Verification items for the finished model (mm, model axes). Coordinates: 2 decimals unless noted, no trailing zeros. Order: outer loops, then holes, each group sorted by start corner. A loop starts at its lowest first (then second) coordinate and runs counter-clockwise, first axis right, second up. Notation, with made-up numbers: M -33.75,29 L 9.25,29 A9 ccw 9.25,45 Z; hole C -31,-10 d3. An arc over 180 degrees is marked long. Return JSON: item names as keys, results as strings.
```python
from build123d import *

# Parameters (mm, degrees)
BOX004_W     = 24
BOX004_H     = 19.8
BOX004_DEPTH = 2
BOX002_W     = 31
BOX002_H     = 45
BOX002_DEPTH = 2
CHAMFER_SIZE = 1


with BuildPart() as topplate_cutout:
    # Box004 → Box004 (new body)
    with BuildSketch(Plane(origin=(-12, 8.6, 5.5), x_dir=(1, 0, 0), z_dir=(0, 0, 1))):
        with Locations((12, 9.9)):
            Rectangle(BOX004_W, BOX004_H)
    extrude(amount=BOX004_DEPTH)


with BuildPart() as topplate:
    # Box002 → Box002 (new body)
    with BuildSketch(Plane(origin=(-15.5, 0, 5.5), x_dir=(1, 0, 0), z_dir=(0, 0, 1))):
        with Locations((15.5, 22.5)):
            Rectangle(BOX002_W, BOX002_H)
    extrude(amount=BOX002_DEPTH)

    # Cut014: cut topPlate_cutout
    add(topplate_cutout.part, mode=Mode.SUBTRACT)

    # Chamfer
    chamfer_edges = [topplate.edges().sort_by_distance(p)[0] for p in [
        (-12, 18.5, 5.5),
        (12, 18.5, 5.5),
    ]]
    chamfer(chamfer_edges, length=CHAMFER_SIZE)


solid = topplate.part
```
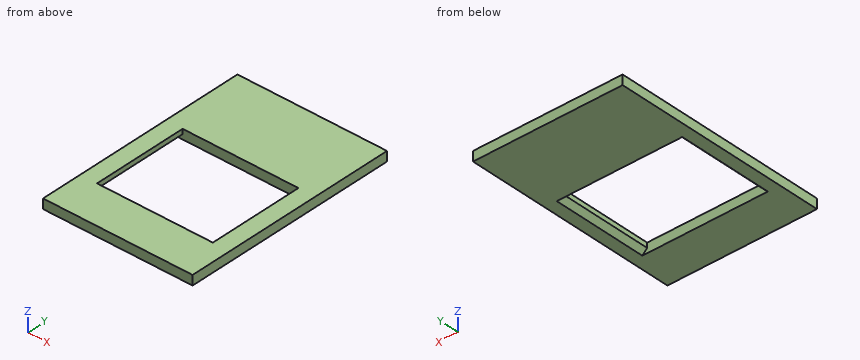
Q1. Cross-section at B-B, the plane z = 5.95. Record the boundary of the cut face in (x, y).
Values:
{"outline": "M -15.5,0 L 15.5,0 L 15.5,45 L -15.5,45 Z; hole M -12.55,8.6 L 12.55,8.6 L 12.55,28.4 L -12.55,28.4 Z"}
Q2. Cross-section at C-C, the plane x = -1.5. Record the boundary of the cut face in (y, z), and give its area (3 significant figures).
Values:
{"outline": "M 0,5.5 L 8.6,5.5 L 8.6,7.5 L 0,7.5 Z; M 28.4,5.5 L 45,5.5 L 45,7.5 L 28.4,7.5 Z", "area": "50.4 mm^2"}
Q3. Material ranges on line 1 along X through (y, z) = (9.5, 6.9); line 2 along Y through (x, z) = (-7, 7.2); line 3 along X through (y, z) = (16, 5.9), recorded low to high.
Values:
{"line 1": "-15.5 to -12, 12 to 15.5", "line 2": "0 to 8.6, 28.4 to 45", "line 3": "-15.5 to -12.6, 12.6 to 15.5"}
Q4. Cross-section at A-A, the plane y = 26.5. Record the boundary of the cut face in (x, z).
Values:
{"outline": "M -15.5,5.5 L -13,5.5 L -12,6.5 L -12,7.5 L -15.5,7.5 Z; M 12,6.5 L 13,5.5 L 15.5,5.5 L 15.5,7.5 L 12,7.5 Z"}
